Geometry check sheet. Reference: the model listing, model coordinates, mm. Round coordinates to 2 decimals unless told otherwise and drop trailing zeros. Loops run counter-clockwise (first coordinate to the right, second up) from the corner with the lowest first, then second, coordinate; pieces in that order, holes last. Notation, with made-up numbers: M 60.25,73 L 105.25,73 A19 cw 105.25,94 Z; hole C 0.25,78.25 d11. An arc over 180 degrees is marked long. Use one line per item in the form item = value. Start each with the question number.
1. Cross-section at C-C (z = 3.5). State how many separate pieces and enclosed holes the cut face has, then the cut area to 3 significant figures.
2. Cross-section at D-D (y = 94.5). Record the boundary of the cut face in (x, z), then the cut area to 3 significant figures.
3. Material ranges on line 1 (X direction, y = 290, z = 6); line 2 (Y direction, x = 10, z = 7.25); line 3 (Y direction, x = 8.5, z = 5.5), recorded low to high.
4. Go/stop test with flat-tipped pins: pin 1 (3.5 mm diameter, centred on x = 70, y = 170, fed in from +Z); pin 2 (3 mm diameter, centred on y = 58, z = 5, fed in from +X); pin 3 (2 mm diameter, centred on y = 226.5, z = 2, fed in from -X). Record where each tip stops, or that it passes through.
5. Cross-section at A-A (x = 40). Record the boundary of the cut face in (y, z), then the cut area to 3 significant figures.
6. Cross-section at B-B (y = 130). Record the boundary of the cut face in (x, z), then the cut area to 3 significant figures.
```python
from build123d import *

# Parameters (mm, degrees)
SKETCH_R   = 2
SKETCH_R_2 = 5
SKETCH_R_3 = 3
PAD_DEPTH  = 10


with BuildPart() as part:
    # Sketch → Pad (new body)
    with BuildSketch(Plane.XY):
        with BuildLine():
            Line((0, 0), (80, 0))
            Line((80, 0), (80, 78.765246))
            ThreePointArc((80, 78.765246), (105, 130), (80, 181.234754))
            Line((80, 181.234754), (80, 350))
            Line((80, 350), (0, 350))
            Line((0, 350), (0, 181.234754))
            ThreePointArc((0, 181.234754), (-25, 130), (0, 78.765246))
            Line((0, 78.765246), (0, 0))
        make_face()
        with Locations((10, 50)):
            Circle(SKETCH_R, mode=Mode.SUBTRACT)
        with Locations((10, 110)):
            Circle(SKETCH_R, mode=Mode.SUBTRACT)
        with Locations((10, 170)):
            Circle(SKETCH_R, mode=Mode.SUBTRACT)
        with Locations((10, 230)):
            Circle(SKETCH_R, mode=Mode.SUBTRACT)
        with Locations((10, 290)):
            Circle(SKETCH_R, mode=Mode.SUBTRACT)
        with Locations((70, 50)):
            Circle(SKETCH_R, mode=Mode.SUBTRACT)
        with Locations((70, 110)):
            Circle(SKETCH_R, mode=Mode.SUBTRACT)
        with Locations((70, 170)):
            Circle(SKETCH_R, mode=Mode.SUBTRACT)
        with Locations((70, 230)):
            Circle(SKETCH_R, mode=Mode.SUBTRACT)
        with Locations((70, 290)):
            Circle(SKETCH_R, mode=Mode.SUBTRACT)
        with Locations((40, 130)):
            Circle(SKETCH_R_2, mode=Mode.SUBTRACT)
        with Locations((40, 205)):
            Circle(SKETCH_R_3, mode=Mode.SUBTRACT)
        with BuildLine():
            ThreePointArc((-1.7193, 171.7193), (-18.943845, 127.426456), (2.075531, 84.803378))
            ThreePointArc((2.075531, 84.803378), (6.302023, 85.173143), (5.932267, 89.399636))
            ThreePointArc((2.52333, 167.476649), (-12.949555, 127.688159), (5.932267, 89.399636))
            ThreePointArc((2.52333, 167.476649), (2.523346, 171.719295), (-1.7193, 171.7193))
        make_face(mode=Mode.SUBTRACT)
        with BuildLine():
            ThreePointArc((74.067734, 89.399637), (92.949555, 127.688158), (77.476671, 167.476648))
            ThreePointArc((81.7193, 171.7193), (77.476654, 171.719295), (77.476671, 167.476648))
            ThreePointArc((77.924469, 84.803378), (98.943845, 127.426456), (81.7193, 171.7193))
            ThreePointArc((74.067734, 89.399637), (73.697977, 85.173144), (77.924469, 84.803378))
        make_face(mode=Mode.SUBTRACT)
    extrude(amount=PAD_DEPTH)


solid = part.part
```
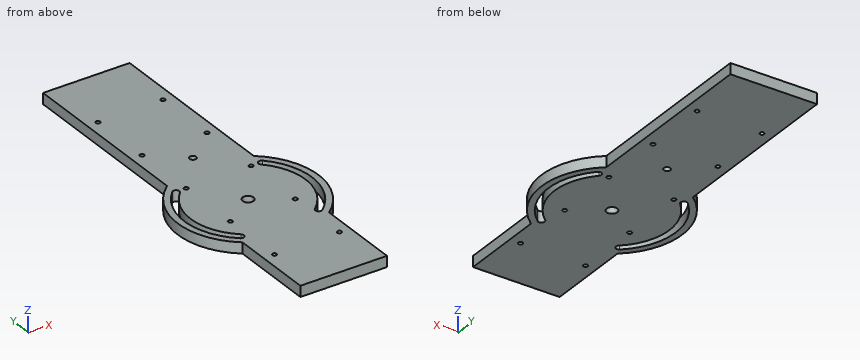
Reported:
q1.separate_pieces = 1
q1.enclosed_holes = 14
q1.area = 30,200 mm²
q2.outline = M -14.45,0 L -7.12,0 L -7.12,10 L -14.45,10 Z; M 0.65,0 L 79.35,0 L 79.35,10 L 0.65,10 Z; M 87.12,0 L 94.45,0 L 94.45,10 L 87.12,10 Z
q2.area = 934 mm²
q3.line_1 = 0 to 8, 12 to 68, 72 to 80
q3.line_2 = 0 to 48, 52 to 108, 112 to 168, 172 to 228, 232 to 288, 292 to 350
q3.line_3 = 0 to 48.68, 51.32 to 108.68, 111.32 to 168.68, 171.32 to 228.68, 231.32 to 288.68, 291.32 to 350
q4.pin_1 = through
q4.pin_2 = 80
q4.pin_3 = 0
q5.outline = M 0,0 L 125,0 L 125,10 L 0,10 Z; M 135,0 L 202,0 L 202,10 L 135,10 Z; M 208,0 L 350,0 L 350,10 L 208,10 Z
q5.area = 3,340 mm²
q6.outline = M -25,0 L -19,0 L -19,10 L -25,10 Z; M -13,0 L 35,0 L 35,10 L -13,10 Z; M 45,0 L 93,0 L 93,10 L 45,10 Z; M 99,0 L 105,0 L 105,10 L 99,10 Z
q6.area = 1,080 mm²
